The model under review builds one solid part; all positions refer to its coordinate system, in mm. A direction names the side the tool comes from. Round coordinates to 2 decimals unless told otherwise and drop trailing zeros. Write each loop counter-clockwise with the first axis right and the second up, starting at its lowest first coordinate (ties: lowest second). Pieces come first, ordered by that corner, then holes. Notation, with made-up numbers: (-30.75, -18.5) - (-1.75, -18.5) arc R34 cw to (-1.75, 19.5) - close; hole circle Ø11 at (22.5, 24.25). An arc over 180 degrees is marked (long way). Return JSON: item names as keys, results as strings.
from build123d import *

# Parameters (mm, degrees)
SKETCH_1_W          = 15
SKETCH_1_H          = 15
SKETCH_1_W_2        = 13
SKETCH_1_H_2        = 13
EXTRUDE_1_DEPTH     = 115
CUT_EXTRUDE_1_DEPTH = 117.216392992


with BuildPart() as part:
    # ｽｹｯﾁ1 → 押し出し-薄板1 (new body)
    with BuildSketch(Plane.XY):
        Rectangle(SKETCH_1_W, SKETCH_1_H)
        Rectangle(SKETCH_1_W_2, SKETCH_1_H_2, mode=Mode.SUBTRACT)
    extrude(amount=EXTRUDE_1_DEPTH)

    # ｽｹｯﾁ2 → ｶｯﾄ - 押し出し1 (cut, through all)
    with BuildSketch(Plane(origin=(0, 7.5, 0), x_dir=(1, 0, 0), z_dir=(0, 1, 0))):
        with BuildLine():
            ThreePointArc((2.1, -110), (1.48492424, -108.51507576), (0, -107.9))
            Line((0, -107.9), (0, -112.1))
            ThreePointArc((0, -112.1), (1.48492424, -111.48492424), (2.1, -110))
        make_face()
        with BuildLine():
            Line((0, -112.1), (0, -107.9))
            ThreePointArc((0, -107.9), (-2.1, -110), (0, -112.1))
        make_face()
        with BuildLine():
            ThreePointArc((2.1, -77.5), (1.48492424, -76.01507576), (0, -75.4))
            Line((0, -75.4), (0, -79.6))
            ThreePointArc((0, -79.6), (1.48492424, -78.98492424), (2.1, -77.5))
        make_face()
        with BuildLine():
            Line((0, -79.6), (0, -75.4))
            ThreePointArc((0, -75.4), (-2.1, -77.5), (0, -79.6))
        make_face()
        with BuildLine():
            Line((0, -57.5), (0, -55.4))
            ThreePointArc((0, -55.4), (-2.1, -57.5), (0, -59.6))
            Line((0, -59.6), (0, -57.5))
        make_face()
        with BuildLine():
            ThreePointArc((2.1, -57.5), (1.48492424, -56.01507576), (0, -55.4))
            Line((0, -55.4), (0, -57.5))
            Line((0, -57.5), (2.1, -57.5))
        make_face()
        with BuildLine():
            Line((2.1, -57.5), (0, -57.5))
            Line((0, -57.5), (0, -59.6))
            ThreePointArc((0, -59.6), (1.48492424, -58.98492424), (2.1, -57.5))
        make_face()
        with BuildLine():
            ThreePointArc((2.1, -37.5), (1.48492424, -36.01507576), (0, -35.4))
            Line((0, -35.4), (0, -39.6))
            ThreePointArc((0, -39.6), (1.48492424, -38.98492424), (2.1, -37.5))
        make_face()
        with BuildLine():
            Line((0, -39.6), (0, -35.4))
            ThreePointArc((0, -35.4), (-2.1, -37.5), (0, -39.6))
        make_face()
        with BuildLine():
            ThreePointArc((2.1, -5), (1.48492424, -3.51507576), (0, -2.9))
            Line((0, -2.9), (0, -7.1))
            ThreePointArc((0, -7.1), (1.48492424, -6.48492424), (2.1, -5))
        make_face()
        with BuildLine():
            Line((0, -7.1), (0, -2.9))
            ThreePointArc((0, -2.9), (-2.1, -5), (0, -7.1))
        make_face()
    extrude(amount=-CUT_EXTRUDE_1_DEPTH, mode=Mode.SUBTRACT)


solid = part.part
(1) Wall thickness on line 1 (Y direction, x = 3.75, z = 19): over which ranges is the line inside the solid? List them lowest first.
Filled in:
{"line 1": "y = -7.5 to -6.5, 6.5 to 7.5"}
(2) Add section B-B (y = 1.5). Write out the cut boundary in (x, z), plus the area to 3 significant figures.
Filled in:
{"outline": "(-7.5, 0) - (-6.5, 0) - (-6.5, 115) - (-7.5, 115) - close; (6.5, 0) - (7.5, 0) - (7.5, 115) - (6.5, 115) - close", "area": "230 mm2"}
(3) Clearance check with a flat-ended pin moving along its axis: pin 1 Ø6 at (x, y) = (-5, -3.5) entering from +Z. State where the tip first meets the part, or that it passes through.
Filled in:
{"pin 1": "stops at z = 115"}
(4) Add section A-A (z = 67). Write out the cut boundary in (x, y).
Filled in:
{"outline": "(-7.5, -7.5) - (7.5, -7.5) - (7.5, 7.5) - (-7.5, 7.5) - close; hole (-6.5, -6.5) - (6.5, -6.5) - (6.5, 6.5) - (-6.5, 6.5) - close"}
(5) Mouldability with a two-part tool opening along X and no side actions: class faces 1 (the flat face through (7.5, 0, 57)), 2 (the flat face through (-7, 0, 115)), 3 (the flat face through (6.5, 0, 57)) as released by +X, released by -X, zero draft, split by the parting line, or undercut.
Filled in:
{"face 1": "released by +X", "face 2": "zero draft", "face 3": "undercut"}
(6) For faces 4 (the flat face through (-3, 6.5, 57)), 5 (the flat face through (-3, 7.5, 57)), list the 3-axis set-ups (+Z, -Z, +X, -X, +Y, -Y) from which the entire face can be reached by the end or side of a thin tool; tool diameter is ignored.
Filled in:
{"face 4": "+Z, -Z", "face 5": "+Z, -Z, +X, -X, +Y"}
